Geometry: final body of the model. Coordinates: model frame, mm. A direction names the side the tool comes from. Coordinates: 2 decimals unless noted, no trailing zeros. Write each loop counter-clockwise with the first axis right and the second up, starting at its lowest first coordinate (ties: lowest second). Pieces come first, ordered by that corner, then holes. Notation, with made-up numbers: (62, -26.75) -> (68, -26.75) arc R25 cw to (68, 12.25) -> close; hole circle Ø5 at (1, 8). An arc over 180 degrees is marked (long way). One line per item, written item: value.
```python
from build123d import *

# Parameters (mm, degrees)
SKETCH1_R           = 9
BOSS_EXTRUDE1_DEPTH = 3
SKETCH2_R           = 2
BOSS_EXTRUDE2_DEPTH = 2
SKETCH3_R           = 1.1
CUT_EXTRUDE1_DEPTH  = 2
SKETCH4_RX          = 3
SKETCH4_RY          = 1
CUT_EXTRUDE2_DEPTH  = 3


with BuildPart() as part:
    # Sketch1 → Boss-Extrude1 (new body)
    with BuildSketch(Plane(origin=(0, 0, 0), x_dir=(1, 0, 0), z_dir=(0, 1, 0))):
        Circle(SKETCH1_R)
    extrude(amount=BOSS_EXTRUDE1_DEPTH)

    # Sketch2 → Boss-Extrude2 (add)
    with BuildSketch(Plane(origin=(0, 3, 0), x_dir=(1, 0, 0), z_dir=(0, 1, 0))):
        Circle(SKETCH2_R)
    extrude(amount=BOSS_EXTRUDE2_DEPTH)

    # Sketch3 → Cut-Extrude1 (cut)
    with BuildSketch(Plane(origin=(0, 5, 0), x_dir=(1, 0, 0), z_dir=(0, 1, 0))):
        Circle(SKETCH3_R)
    extrude(amount=-CUT_EXTRUDE1_DEPTH, mode=Mode.SUBTRACT)

    # Sketch4 → Cut-Extrude2 (cut)
    with BuildSketch(Plane(origin=(0, 3, 0), x_dir=(1, 0, 0), z_dir=(0, 1, 0))):
        with Locations(Location((0, 5.49925853), (0, 0, 90))):
            Ellipse(SKETCH4_RX, SKETCH4_RY)
    extrude(amount=-CUT_EXTRUDE2_DEPTH, mode=Mode.SUBTRACT)


solid = part.part
```
(1) Section C-C (x = -1.5). Return the cut outline in (y, z), then the cut area to 3 significant figures.
Responses:
outline: (0, -8.87) -> (3, -8.87) -> (3, -1.32) -> (5, -1.32) -> (5, 1.32) -> (3, 1.32) -> (3, 8.87) -> (0, 8.87) -> close
area: 58.5 mm2
(2) Section A-A (z = 0). Return the cut outline in (x, y).
Responses:
outline: (-9, 0) -> (9, 0) -> (9, 3) -> (2, 3) -> (2, 5) -> (1.1, 5) -> (1.1, 3) -> (-1.1, 3) -> (-1.1, 5) -> (-2, 5) -> (-2, 3) -> (-9, 3) -> close
(3) Pull-direction query (Z, two-part tool) for faces 3 (the flat face through (1, 5, 1)), 4 (the flat face through (0, 3, 0)), 5 (the cylindrical face through (-1.172, 1.479, -8.923)); classes: released by +Z, released by -Z, zero draft, split by the parting line, or undercut.
Responses:
face 3: zero draft
face 4: undercut
face 5: split by the parting line
(4) Reachability of faces 1 (the cylindrical face through (1.05, 4.01, -0.33)), 2 (the flat face through (0, 0, 0)) from +Z, -Z, +X, -X, +Y, -Y: full face, straight path, thin tool, end or side. Return the list, or none.
Responses:
face 1: +Y
face 2: +Z, -Z, +X, -X, -Y
(5) First-contact query: pin 1 (3 mm diameter, centred on x = 6.5, z = -3.5, fed in from -Y); pin 2 (1.5 mm diameter, centred on y = 0.5, z = -4, fed in from -X); pin 3 (0.7 mm diameter, centred on x = -0.5, z = -0.5, fed in from +Y); pin 4 (1 mm diameter, centred on y = 2, z = 1, fed in from -X). Flat tips, straight axial feed; report the tip coordinate or a pass-through.
Responses:
pin 1: stops at y = 0
pin 2: stops at x = -8.39
pin 3: stops at y = 3
pin 4: stops at x = -8.99
(6) Section D-D (x = -6). Return the cut outline in (y, z), then the cut area to 3 significant figures.
Responses:
outline: (0, -6.71) -> (3, -6.71) -> (3, 6.71) -> (0, 6.71) -> close
area: 40.2 mm2
(7) Section B-B (y = 3.25). Return the cut outline in (x, z).
Responses:
outline: circle Ø4 at (0, 0); hole circle Ø2.2 at (0, 0)
(8) Line query: line 1 (X direction, y = 4.6, z = 0); line 2 (Y direction, x = 1, z = 6.75). Output: solid intervals per line, ascending. Write a range as [from, to].
Responses:
line 1: x = [-2, -1.1], [1.1, 2]
line 2: y = [0, 3]
